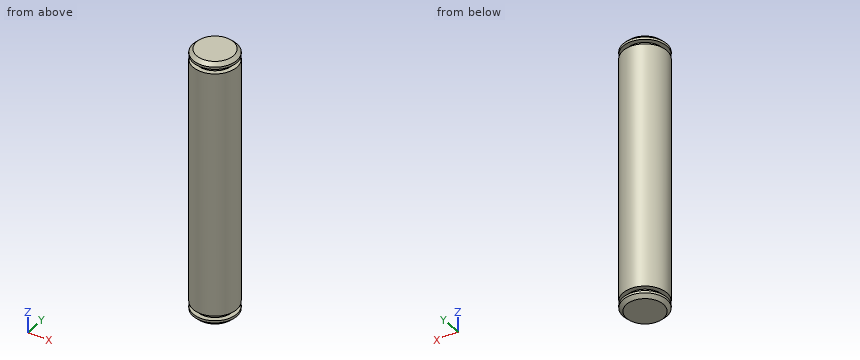
from build123d import *

# Parameters (mm, degrees)
ESQUISSE1_R                = 9.5
BASE_EXTRUSION_DEPTH       = 116
CHANFREIN1_SIZE            = 1.5
ESQUISSE2_R                = 12
ESQUISSE2_R_2              = 7.5
ENL_V_MAT_EXTRU_1_DEPTH    = 2
R_P_TITION_LIN_AIRE1_COUNT = 2
R_P_TITION_LIN_AIRE1_PITCH = 109


with BuildPart() as part:
    # Esquisse1 → Base-Extrusion (new body)
    with BuildSketch(Plane.XY):
        with Locations(Location((0, 0, 0), (0, 0, 180))):
            Circle(ESQUISSE1_R)
    extrude(amount=BASE_EXTRUSION_DEPTH)

    # Chanfrein1
    chanfrein1_edges = [part.edges().sort_by_distance(p)[0] for p in [
        (9.5, 0, 0),
        (9.5, 0, 116),
    ]]
    chamfer(chanfrein1_edges, length=CHANFREIN1_SIZE)

    # Esquisse2 → Enlèv. mat.-Extru.1 (cut)
    with BuildSketch(Plane.XY.offset(113.5)):
        Circle(ESQUISSE2_R)
        Circle(ESQUISSE2_R_2, mode=Mode.SUBTRACT)
    enl_v_mat_extru_1 = extrude(amount=-ENL_V_MAT_EXTRU_1_DEPTH, mode=Mode.SUBTRACT)

    # Répétition linéaire1: Enlèv. mat.-Extru.1 ×2
    with Locations(*[(0, 0, -i * R_P_TITION_LIN_AIRE1_PITCH) for i in range(1, R_P_TITION_LIN_AIRE1_COUNT)]):
        add(enl_v_mat_extru_1, mode=Mode.SUBTRACT)


solid = part.part
Source: CAD feature listing. Evaluate the final solid. Frame: model axes, mm. Coordinates: 2 decimals unless noted, no trailing zeros. Order: outer loops, then holes, each group sorted by start corner. A loop starts at its lowest first (then second) coordinate and runs counter-clockwise, first axis right, second up. Notation, with made-up numbers: M -26,6 L 14,6 A20 ccw 14,45 Z; hole C 81,28 d4. An arc over 180 degrees is marked long. Write each question's results on one line, items separated by ' | '. Start each with the question number.
1. Section A-A, the plane z = 93.5. Return the cut outline in (x, y).
2. Pin query (flat end, axial travel): pin 1 (10 mm diameter, centred on x = -7.5, z = 18.5, fed in from +Y). Return the tip coordinate at first contact, or that it passes through.
3. Material intervals for L1, parallel to Z at x = -7.75, y = 1.25; L2, parallel to Z at x = -7, y = -5.25; L3, parallel to Y at x = -0.5, z = 16, sorted ascending.
Solution:
1) outline: C 0,0 d19
2) pin 1: y = 9.17
3) L1: 0 to 2.5, 4.5 to 111.5, 113.5 to 116 | L2: 0.75 to 2.5, 4.5 to 111.5, 113.5 to 115.25 | L3: -9.49 to 9.49
